```python
from build123d import *

# Parameters (mm, degrees)
F0_R     = 1.5
F1_DEPTH = 3
F0_R_2   = 3
F2_DEPTH = 3
F4_D     = 3


with BuildPart() as f1:
    # F0 (on Front) → F1 (new body)
    with BuildSketch(Plane.XZ):
        with BuildLine():
            Line((-57.8970168753, 22.2757457812), (-75, 18))
            ThreePointArc((-75, 18), (-72.1715728753, 16.8284271247), (-71, 14))
            ThreePointArc((-71, 14), (-72.1715728753, 11.1715728753), (-75, 10))
            Line((-75, 10), (-56.6075588533, 9.2336482856))
            ThreePointArc((-56.6075588533, 9.2336482856), (-56.0921877833, 15.8693948691), (-57.8970168753, 22.2757457812))
        make_face()
        with BuildLine():
            Line((-51, 24), (-57.8970168753, 22.2757457812))
            ThreePointArc((-57.8970168753, 22.2757457812), (-56.0921877833, 15.8693948691), (-56.6075588533, 9.2336482856))
            Line((-56.6075588533, 9.2336482856), (-51, 9))
            Line((-51, 9), (-50, 6.5993144652))
            Line((-50, 6.5993144652), (-42, 6.5993144652))
            Line((-42, 6.5993144652), (-36.7907804817, 4.091785901))
            ThreePointArc((-36.7907804817, 4.091785901), (-30.7, 5.3517437692), (-24.6092195183, 4.091785901))
            Line((-24.6092195183, 4.091785901), (-19.4, 6.5993144652))
            Line((-19.4, 6.5993144652), (-11.4, 6.5993144652))
            Line((-11.4, 6.5993144652), (-10.2805419503, 9))
            Line((-10.2805419503, 9), (10.2805419503, 9))
            Line((10.2805419503, 9), (11.4, 6.5993144652))
            Line((11.4, 6.5993144652), (19.4, 6.5993144652))
            Line((19.4, 6.5993144652), (24.6092195183, 4.091785901))
            ThreePointArc((24.6092195183, 4.091785901), (30.7, 5.3517437692), (36.7907804817, 4.091785901))
            Line((36.7907804817, 4.091785901), (42, 6.5993144652))
            Line((42, 6.5993144652), (50, 6.5993144652))
            Line((50, 6.5993144652), (51, 9))
            Line((51, 9), (56.6075588533, 9.2336482856))
            ThreePointArc((56.6075588533, 9.2336482856), (56.0921877833, 15.8693948691), (57.8970168753, 22.2757457812))
            Line((57.8970168753, 22.2757457812), (51, 24))
            Line((51, 24), (45.6189500386, 24))
            ThreePointArc((45.6189500386, 24), (38.5092844997, 9.8794625444), (23.5729752888, 15.0605424767))
            Line((23.5729752888, 15.0605424767), (0, 12.9805740689))
            Line((0, 12.9805740689), (-23.5729752888, 15.0605424767))
            ThreePointArc((-23.5729752888, 15.0605424767), (-38.5092844997, 9.8794625444), (-45.6189500386, 24))
            Line((-45.6189500386, 24), (-51, 24))
        make_face()
        Polygon((-20.2601172091, 24), (-23.5729752888, 15.0605424767), (0, 12.9805740689), (23.5729752888, 15.0605424767), (20.2601172091, 24), (4.7092107675, 24), (0.9159085684, 21.9222409377), (-0.9159085684, 21.9222409377), (-4.7092107675, 24), align=None)
        with Locations((0, 18)):
            Circle(F0_R, mode=Mode.SUBTRACT)
        with BuildLine():
            Line((73.569615724, 21.8710863814), (57.8970168753, 22.2757457812))
            ThreePointArc((57.8970168753, 22.2757457812), (56.0921877833, 15.8693948691), (56.6075588533, 9.2336482856))
            Line((56.6075588533, 9.2336482856), (83, 9.2336482856))
            Line((83, 9.2336482856), (83, 21.8710863814))
            Line((83, 21.8710863814), (73.569615724, 21.8710863814))
        make_face()
        with Locations((75, 14)):
            Circle(F0_R, mode=Mode.SUBTRACT)
        with BuildLine():
            ThreePointArc((36.7907804817, 4.091785901), (30.7, 5.3517437692), (24.6092195183, 4.091785901))
            Line((24.6092195183, 4.091785901), (28.2, -10))
            ThreePointArc((28.2, -10), (30.7, -12.5), (33.2, -10))
            Line((33.2, -10), (36.7907804817, 4.091785901))
        make_face()
        with Locations((30.7, -10)):
            Circle(F0_R, mode=Mode.SUBTRACT)
        with BuildLine():
            ThreePointArc((-24.6092195183, 4.091785901), (-30.7, 5.3517437692), (-36.7907804817, 4.091785901))
            Line((-36.7907804817, 4.091785901), (-33.2, -10))
            ThreePointArc((-33.2, -10), (-30.7, -12.5), (-28.2, -10))
            Line((-28.2, -10), (-24.6092195183, 4.091785901))
        make_face()
        with Locations((-30.7, -10)):
            Circle(F0_R, mode=Mode.SUBTRACT)
    extrude(amount=F1_DEPTH)

    # F0 (on Front) → F2 (join, symmetric)
    with BuildSketch(Plane.XZ):
        with BuildLine():
            ThreePointArc((-71, 14), (-72.1715728753, 16.8284271247), (-75, 18))
            ThreePointArc((-75, 18), (-79, 14), (-75, 10))
            ThreePointArc((-75, 10), (-72.1715728753, 11.1715728753), (-71, 14))
        make_face()
        with Locations((-75, 14)):
            Circle(F0_R_2, mode=Mode.SUBTRACT)
    extrude(amount=F2_DEPTH, both=True)

    # F4 (through all)
    with Locations(Plane.XZ.offset(3)):
        with Locations((-51, 20), (51, 20)):
            Hole(F4_D / 2)


solid = f1.part
```
Geometry check sheet. Reference: the model listing, model coordinates, mm. A direction names the side the tool comes from. Give positions to 0.01 mm unless a question says otherwise; leave off trailing zeros. Write each loop counter-clockwise with the first axis right and the second up, starting at its lowest first coordinate (ties: lowest second). Pieces come first, ordered by that corner, then holes. Notation, with made-up numbers: (-7, 85.5) - (15, 85.5) arc R18 cw to (15, 107.5) - close; hole circle Ø1 at (87, -1). An arc over 180 degrees is marked (long way). Use a Markdown table: item, result.
Q1. Set-up check for faces 4 (the face through (-46, -1, 6.599)), 5 (the face through (21.97, -1.48, 5.36)), 6 (the face through (39.36, -1.48, 5.33)): record each of +Z, -Z, +X, -X, +Y, -Y from which the full face is reachable in a straight line by a thin tool's end or side.
Computed:
| item | result |
|---|---|
| face 4 | -Z, -X, +Y, -Y |
| face 5 | -Z, +Y, -Y |
| face 6 | -Z, +X, +Y, -Y |
Q2. Section check B-B, the plane x = 8. Enter the section's corners in (y, z).
Computed:
| item | result |
|---|---|
| outline | (-3, 9) - (0, 9) - (0, 24) - (-3, 24) - close |
Q3. Section check C-C, the plane x = -66.5. Enter the section's corners in (y, z) (3 decimals).
Computed:
| item | result |
|---|---|
| outline | (-3, 9.646) - (0, 9.646) - (0, 20.125) - (-3, 20.125) - close |
Q4. Go/stop test with flat-tipped pins: P1, Ø2, axis at x = -10.5, y = 1.5, coming from the +Z side; P2, Ø2, axis at x = 0, y = -2, coming from the +Z side; P3, Ø3, axis at y = 1, z = 12, coming from the +X side; P4, Ø4, axis at x = 0, z = 18, coming from the +Y side. Record where each tip stops, or that it passes through.
Computed:
| item | result |
|---|---|
| P1 | passes through |
| P2 | stops at z = 21.97 |
| P3 | stops at x = 83 |
| P4 | stops at y = 0 |
Q5. Draft check along Z on faces 1 (the face through (-2.79, -1.48, 22.95)), 2 (the face through (-38.28, -1.48, 9.79)), 3 (the face through (46, -1, 6.599)). Enter one of: pulls with the +Z half, pulls with the -Z half, needs draft (parallel to the pull), parting line crosses it, or undercut.
Computed:
| item | result |
|---|---|
| face 1 | pulls with the +Z half |
| face 2 | undercut |
| face 3 | pulls with the -Z half |
Q6. Thickness scan on L1, parallel to Z at x = -51, y = -1.95; L2, parallel to X at y = -0.1, z = 16; L3, parallel to Z at x = 72, y = -1. Record the ranges inside material, lowest first. Write a range as [from, to].
Computed:
| item | result |
|---|---|
| L1 | z = [9, 18.5], [21.5, 24] |
| L2 | x = [-78.46, -77.24], [-72.76, -44.91], [-23.22, 23.22], [44.91, 83] |
| L3 | z = [9.23, 21.91] |
Q7. Section check A-A, the plane y = 1.5. Enter the section's corners in (x, z), then the cut area to 3 significant figures.
Computed:
| item | result |
|---|---|
| outline | circle Ø8 at (-75, 14); hole circle Ø6 at (-75, 14) |
| area | 22.0 mm² |
